Autodesk Inventor part; units mm, degrees
ref_plane "YZ Plane" through (0, 0, 0) normal (1, 0, 0) x (0, 1, 0)
ref_plane "XZ Plane" through (0, 0, 0) normal (0, 1, 0) x (-1, 0, 0)
ref_plane "XY Plane" through (0, 0, 0) normal (0, 0, 1) x (1, 0, 0)
sketch "Szkic1" plane through (0, 0, 0) normal (0, 0, 1) x (1, 0, 0)
  line L0 (10.5195, 87.461) -> (10.5195, -76.7273)
  line L1 (-15.4805, 77.7078) -> (-89.4805, 77.7078)
  line L2 (-89.4805, 77.7078) -> (-89.4805, 74.7078)
  line L3 (-89.4805, 74.7078) -> (-18.4805, 74.7078)
  line L4 (-18.4805, 74.7078) -> (-18.4805, 15.7078)
  line L5 (-18.4805, 15.7078) -> (-89.4805, 15.7078)
  line L6 (-89.4805, 15.7078) -> (-89.4805, 12.7078)
  line L7 (-89.4805, 12.7078) -> (-15.4805, 12.7078)
  line L8 (-15.4805, 77.7078) -> (-15.4805, 12.7078)
  point P0 (0, 0)
  dimension "d0" = 65
  dimension "d1" = 52
  dimension "d2" = 58
  dimension "d3" = 3
  dimension "d4" = 3
  dimension "d5" = 200
revolve "Obrót1" add sketch "Szkic1" angle 360 about axis through (10.5195, 87.461, 0) along (0, -1, 0)
properties part number "szpula"
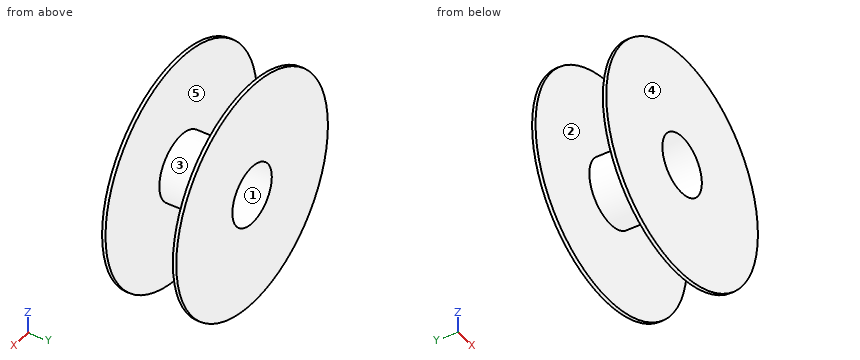
The model under review builds one solid part; all positions refer to its coordinate system, in mm. Face numbers are marked on the shaded views. A direction names the side the tool comes from. Give positions to 0.01 mm unless a question says otherwise; leave off trailing zeros. Write each loop counter-clockwise with the first axis right and the second up, starting at its lowest first coordinate (ties: lowest second). Pieces come first, ordered by that corner, then holes. Notation, with made-up numbers: (86.25, -32.75) - (100.25, -32.75) arc R16 ccw to (100.25, -2.75) - close; hole circle Ø1 at (9, 17). An arc over 180 degrees is marked (long way). Answer in a Markdown table with one row per item. Add a question column.
1. We need section B-B on x = 24. Write out the cut boundary in (y, z).
2. Draft analysis for pull direction X (two halves, no side actions). For the marked faces 1, 2 and 3, state which applies: +X half, -X half, draft (parallel to the pull), parting line (faces both ways), or undercut.
3. We need section D-D on y = 50.5. Write out the cut boundary in (x, z).
4. We need section A-A on z = 0. Write out the cut boundary in (x, y), then the cut area to 3 significant figures.
5. Tool access review of the marked faces 4 and 5: name each direction out of +Z, -Z, +X, -X, +Y, -Y from which nothing blocks a thin tool from reaching the whole face with its end or side.
6. Insertion check: P1, Ø6, axis at y = 48, z = 18.5, coming from the -X side; P2, Ø10, axis at x = 13.5, y = 69.5, coming from the +Z side; P3, Ø2, axis at x = 36.5, y = 33, coming from the -Z side. Each pin has a flat end and moves straight along its axis. Give the tip position at first contact, or say it passes through.
7. Wall thickness on line 1 along Y through (x, z) = (62.5, 4); line 2 along X through (y, z) = (27, 0); line 3 along X through (y, z) = (28, -11.5): over which ranges is each line inside the solid? List them lowest first. Write a range as [from, to].
8. We need section C-C on z = -85. Write out the cut boundary in (x, y), then the cut area to 3 significant figures.
Ans:
| question | item | result |
|---|---|---|
| 1 | outline | (12.71, -99.09) - (15.71, -99.09) - (15.71, -25.68) - (74.71, -25.68) - (74.71, -99.09) - (77.71, -99.09) - (77.71, -22.23) - (12.71, -22.23) - close; (12.71, 22.23) - (77.71, 22.23) - (77.71, 99.09) - (74.71, 99.09) - (74.71, 25.68) - (15.71, 25.68) - (15.71, 99.09) - (12.71, 99.09) - close |
| 2 | face 1 | undercut |
| 2 | face 2 | draft |
| 2 | face 3 | parting line |
| 3 | outline | circle Ø58 at (10.52, 0); hole circle Ø52 at (10.52, 0) |
| 4 | outline | (-89.48, 12.71) - (-15.48, 12.71) - (-15.48, 77.71) - (-89.48, 77.71) - (-89.48, 74.71) - (-18.48, 74.71) - (-18.48, 15.71) - (-89.48, 15.71) - close; (36.52, 12.71) - (110.52, 12.71) - (110.52, 15.71) - (39.52, 15.71) - (39.52, 74.71) - (110.52, 74.71) - (110.52, 77.71) - (36.52, 77.71) - close |
| 4 | area | 1,240 mm^2 |
| 5 | face 4 | +Z, -Z, +X, -X, -Y |
| 5 | face 5 | none |
| 6 | P1 | stops at x = -13.99 |
| 6 | P2 | stops at z = 29 |
| 6 | P3 | stops at z = -14.73 |
| 7 | line 1 | y = [12.71, 15.71], [74.71, 77.71] |
| 7 | line 2 | x = [-18.48, -15.48], [36.52, 39.52] |
| 7 | line 3 | x = [-16.1, -12.8], [33.84, 37.14] |
| 8 | outline | (-42.16, 12.71) - (63.2, 12.71) - (63.2, 15.71) - (-42.16, 15.71) - close; (-42.16, 74.71) - (63.2, 74.71) - (63.2, 77.71) - (-42.16, 77.71) - close |
| 8 | area | 632 mm^2 |
